```python
from build123d import *

# Parameters (mm, degrees)
SKETCH5_R             = 3.175
CUT_EXTRUDE1_DEPTH    = 45.676210112
F_2_56_TAPPED_HOLE1_D = 1.778


with BuildPart() as part:
    # Sketch1 → Revolve1 (revolve)
    with BuildSketch(Plane.XY, mode=Mode.PRIVATE) as revolve1_sk:
        Polygon((0, -22.225), (2.38125, -22.225), (3.175, -21.43125), (3.175, 21.43125), (2.38125, 22.225), (0, 22.225), align=None)
    revolve(revolve1_sk.sketch.rotate(Axis((0, -22.225, 0), (0, 1, 0)), 90), axis=Axis((0, -22.225, 0), (0, 1, 0)))

    # Sketch5 → Cut-Extrude1 (cut, through all)
    with BuildSketch(Plane(origin=(0, 22.225, 0), x_dir=(1, 0, 0), z_dir=(0, 1, 0))):
        Circle(SKETCH5_R)
        Polygon((2.38125, -1.374815329), (2.38125, 1.374815329), (0, 2.749630657), (-2.38125, 1.374815329), (-2.38125, -1.374815329), (0, -2.749630657), align=None, mode=Mode.SUBTRACT)
    extrude(amount=-CUT_EXTRUDE1_DEPTH, mode=Mode.SUBTRACT)

    # #2-56 Tapped Hole1 (through all)
    with Locations(Plane(origin=(0, -22.225, 0), x_dir=(-1, 0, 0), z_dir=(0, -1, 0))):
        with Locations((0, 0)):
            Hole(F_2_56_TAPPED_HOLE1_D / 2)


solid = part.part
```
The model under review builds one solid part; all positions refer to its coordinate system, in mm. Coordinates: 2 decimals unless noted, no trailing zeros. Write each loop counter-clockwise with the first axis right and the second up, starting at its lowest first coordinate (ties: lowest second). Pieces come first, ordered by that corner, then holes. Notation, with made-up numbers: (9, 73) -> (59, 73) arc R11 cw to (59, 85) -> close; hole circle Ø4 at (55.25, 31.25). An arc over 180 degrees is marked (long way). One line per item, written item: value. Start each with the question number.
Q1. The part is to be moulded in two halves that separate along Z. For faces 1 (the face through (2.172, -22.095, 1.261)), 2 (the face through (2.2, 22.1, -1.2)), 3 (the face through (-0.19, 0.31, 0.87)), 4 (the face through (1, -22.225, 0.5)), say which applies: +Z half, -Z half, draft (parallel to the pull), parting line (faces both ways), or undercut.
Q2. Add section A-A, the plane y = -3. Give the boundary of the cut face in (x, z), then the cut area to 3 significant figures.
Q3. To check wall thickness, follow probe 1 along Z at (x, y) = (-0.1, -7); probe 2 along Z at (x, y) = (0.4, 15); probe 3 along Z at (x, y) = (-2, 4). State the ranges of each line that lie inside material, in increasing order.
Q4. Clearance check with flat-ended pins moving along their axes: P1, Ø2, axis at x = -1.5, y = -7.5, coming from the -Z side; P2, Ø1, axis at x = 2, y = -8, coming from the -Z side. State where each tip first meets the part, or that it passes through.
Response:
1. face 1: +Z half
1. face 2: -Z half
1. face 3: undercut
1. face 4: draft
2. outline: (-2.38, -1.37) -> (0, -2.75) -> (2.38, -1.37) -> (2.38, 1.37) -> (0, 2.75) -> (-2.38, 1.37) -> close; hole circle Ø1.78 at (0, 0)
2. area: 17.2 mm²
3. probe 1: -2.69 to -0.88, 0.88 to 2.69
3. probe 2: -2.52 to -0.79, 0.79 to 2.52
3. probe 3: -1.59 to 1.59
4. P1: z = -2.46
4. P2: z = -1.88
